Job drawing, mm, ordinate dimensions from the low corner. One solid piece. A direction names the side the tool comes from. Coordinates: 2 decimals unless noted, no trailing zeros. Loops run counter-clockwise (first coordinate to the right, second up) from the corner with the lowest first, then second, coordinate; pieces in that order, holes last. Notation, with made-up numbers: (51.25, -34.75) - (72.25, -34.75) arc R17 cw to (72.25, -5.75) - close; hole circle Ø9 at (78.5, 84.5). An arc over 180 degrees is marked (long way). One line per question, with ' | ' between items. Start each with the question number.
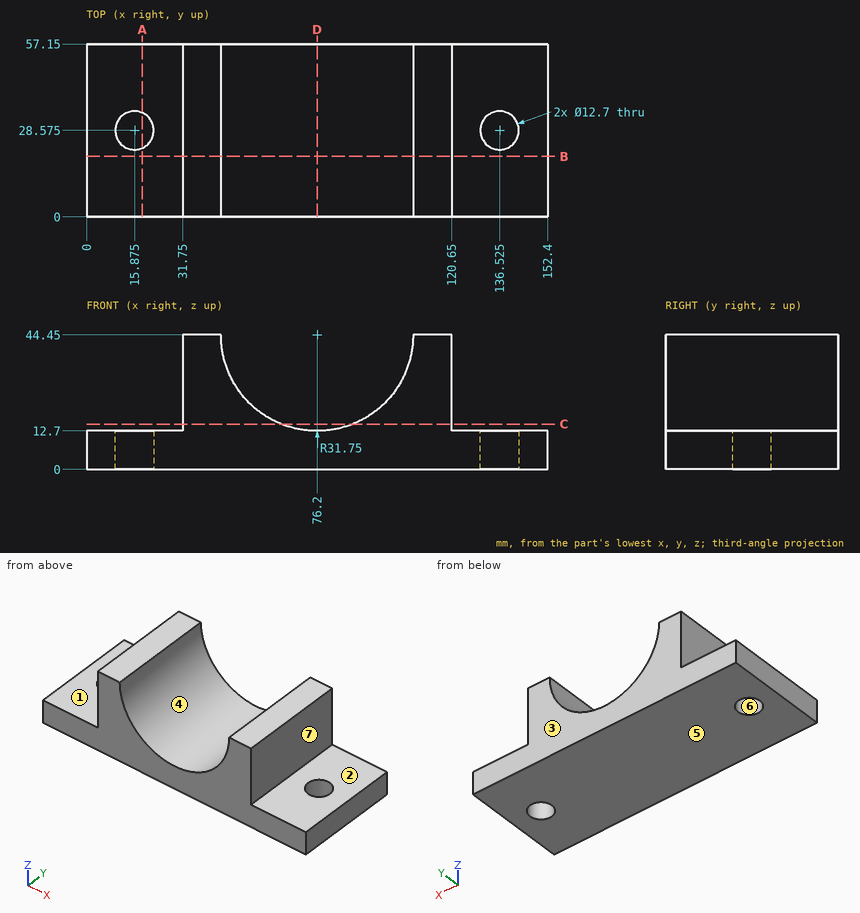
1) Band-saw the part on D-D on x = 76.2. List the corners of the cut face in (y, z).
2) Band-saw the part on A-A on x = 18.5. List the corners of the cut face in (y, z), then the cut area to 3 significant figures.
3) Mould opens along X. For the marked faces 4, 5, 6 and 7 say: +X half, -X half, draft (parallel to the pull), parting line (faces both ways), or undercut.
4) Pin check, flat tips, straight feed: pin 1 Ø3 at (x, y) = (23.5, 32) entering from +Z; pin 2 Ø8 at (y, z) = (45.5, 27.5) entering from +X; pin 3 Ø2 at (y, z) = (38.5, 17.5) entering from -X; pin 4 Ø7.5 at (x, y) = (15.875, 28.575) entering from -Z. Stop position of each tip, or through.
5) Wall check: line 1 along X through (y, z) = (27, 6); line 2 along Z through (x, y) = (10.5, 5.5); line 3 along X through (y, z) = (14.5, 30.5). Give the ranges that are in metal, low to high. Write a range as [from, to].
6) Band-saw the part on B-B on y = 20. List the corners of the cut face in (x, z).
7) Band-saw the part on C-C on z = 15. List the corners of the cut face in (x, y), then the cut area to 3 significant figures.
8) Tool access for the marked faces 1, 2 and 3: list every direction of +Z, -Z, +X, -X, +Y, -Y with a clear straight run to the whole face (end or side of a thin tool).
Values found:
1) outline: (0, 0) - (57.15, 0) - (57.15, 12.7) - (0, 12.7) - close
2) outline: (0, 0) - (22.79, 0) - (22.79, 12.7) - (0, 12.7) - close; (34.36, 0) - (57.15, 0) - (57.15, 12.7) - (34.36, 12.7) - close | area: 579 mm²
3) face 4: undercut | face 5: draft | face 6: undercut | face 7: +X half
4) pin 1: z = 12.7 | pin 2: x = 120.65 | pin 3: x = 31.75 | pin 4: through
5) line 1: [0, 9.72], [22.03, 130.37], [142.68, 152.4] | line 2: [0, 12.7] | line 3: [31.75, 47.68], [104.72, 120.65]
6) outline: (0, 0) - (152.4, 0) - (152.4, 12.7) - (120.65, 12.7) - (120.65, 44.45) - (107.95, 44.45) arc R31.75 cw to (44.45, 44.45) - (31.75, 44.45) - (31.75, 12.7) - (0, 12.7) - close
7) outline: (31.75, 0) - (64.34, 0) - (64.34, 57.15) - (31.75, 57.15) - close; (88.06, 0) - (120.65, 0) - (120.65, 57.15) - (88.06, 57.15) - close | area: 3,720 mm²
8) face 1: +Z, -X, +Y, -Y | face 2: +Z, +X, +Y, -Y | face 3: +Z, -Z, +X, -X, +Y
